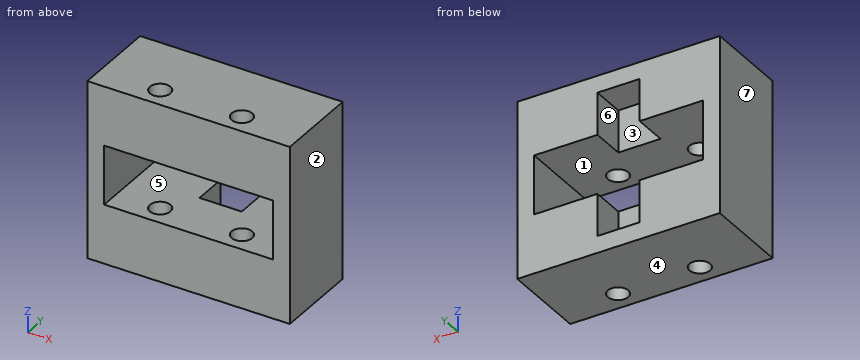
```python
from build123d import *

# Parameters (mm, degrees)
ESQUISSE2_R        = 1.225
BOSS_EXTRU_1_DEPTH = 7
ESQUISSE3_W        = 5
ESQUISSE3_H        = 4
BOSS_EXTRU_2_DEPTH = 2
ESQUISSE5_W        = 2
ESQUISSE5_H        = 10.15
BOSS_EXTRU_3_DEPTH = 7


with BuildPart() as part:
    # Esquisse2 → Boss.-Extru.1 (new body)
    with BuildSketch(Plane.XY):
        Polygon((12, 5.075), (2.5, 5.075), (2.5, 1.075), (-2.5, 1.075), (-2.5, 5.075), (-12, 5.075), (-12, -5.075), (12, -5.075), align=None)
        with Locations((4.845, -2.675)):
            Circle(ESQUISSE2_R, mode=Mode.SUBTRACT)
        with Locations((-4.845, -2.675)):
            Circle(ESQUISSE2_R, mode=Mode.SUBTRACT)
    extrude(amount=BOSS_EXTRU_1_DEPTH)

    # Esquisse3 → Boss.-Extru.2 (add)
    with BuildSketch(Plane.XY.offset(7)):
        with Locations((0, 3.075)):
            Rectangle(ESQUISSE3_W, ESQUISSE3_H)
    extrude(amount=-BOSS_EXTRU_2_DEPTH)

    # Esquisse5 → Boss.-Extru.3 (add)
    with BuildSketch(Plane(origin=(0, 0, 0), x_dir=(-1, 0, 0), z_dir=(0, 0, -1))):
        with Locations((-11, 0)):
            Rectangle(ESQUISSE5_W, ESQUISSE5_H)
        with Locations((11, 0)):
            Rectangle(ESQUISSE5_W, ESQUISSE5_H)
    extrude(amount=BOSS_EXTRU_3_DEPTH)

    # Symétrie1: part across plane


with BuildPart() as part_1:
    add(part.part)
    add(part.part.mirror(Plane(origin=(0, 0, -3.5), x_dir=(1, 0, 0), z_dir=(0, 0, -1))))


solid = part_1.part
```
Can you work these out from the model? Positions are in its coordinate system, mm. Face numbers are marked on the shaded views. A direction names the side the tool comes from. Coordinates: 2 decimals unless noted, no trailing zeros. Order: outer loops, then holes, each group sorted by start corner. A loop starts at its lowest first (then second) coordinate and runs counter-clockwise, first axis right, second up.
1. I'm going to push a flat-ended pin straight in: pin 1 (1.5 mm diameter, centred on x = -0.5, z = -10, fed in from +Y) (3 decimals). Where does the tip first touch, or does it pass through?
2. Thinking about a two-plate mould opening in X: for the marked faces 1, 2, 3 and 4, which applies, +X half, -X half, draft (parallel to the pull), parting line (faces both ways), or undercut?
3. If we section it at B-B (x = -1.5): Please give me the cut outline in (y, z) (3 decimals).
4. If we section it at C-C (y = 3.25): Please give me the cut outline in (x, z).
5. For the marked faces 5, 6 and 7, which set-ups out of +Z, -Z, +X, -X, +Y, -Y let a thin tool reach every point of the face, with its end or its side?
6. If we section it at D-D (x = -5): Please give me the cut outline in (y, z) (3 decimals).
7. I need wall thicknesses on line 1 (X direction, y = 1, z = -4); line 2 (Z direction, x = 2.75, y = 1); line 3 (X direction, y = 2.5, z = -7.75). Which ranges of each line are inside material? Lowest first, please.
8. If we section it at A-A (z = -3.25): Please give me the cut outline in (x, y) (3 decimals).
Entries:
1. pin 1: stops at y = 1.075
2. face 1: undercut
2. face 2: +X half
2. face 3: undercut
2. face 4: draft
3. outline: (-5.075, -14) - (5.075, -14) - (5.075, -12) - (1.075, -12) - (1.075, -7) - (-5.075, -7) - close; (-5.075, 0) - (1.075, 0) - (1.075, 5) - (5.075, 5) - (5.075, 7) - (-5.075, 7) - close
4. outline: (-12, -14) - (12, -14) - (12, 7) - (-12, 7) - close; hole (-10, -7) - (-2.5, -7) - (-2.5, -12) - (2.5, -12) - (2.5, -7) - (10, -7) - (10, 0) - (2.5, 0) - (2.5, 5) - (-2.5, 5) - (-2.5, 0) - (-10, 0) - close
5. face 5: +Y, -Y
5. face 6: +Y
5. face 7: +Z, -Z, -X, +Y, -Y
6. outline: (-5.075, -14) - (-3.89, -14) - (-3.89, -7) - (-5.075, -7) - close; (-5.075, 0) - (-3.89, 0) - (-3.89, 7) - (-5.075, 7) - close; (-1.46, -14) - (5.075, -14) - (5.075, -7) - (-1.46, -7) - close; (-1.46, 0) - (5.075, 0) - (5.075, 7) - (-1.46, 7) - close
7. line 1: x = -12 to -10, 10 to 12
7. line 2: z = -14 to -7, 0 to 7
7. line 3: x = -12 to -2.5, 2.5 to 12
8. outline: (-12, -5.075) - (-10, -5.075) - (-10, 5.075) - (-12, 5.075) - close; (10, -5.075) - (12, -5.075) - (12, 5.075) - (10, 5.075) - close
